For this review, take the finished solid that the model builds, in its own axes (mm). Face numbers are marked on the shaded views. A direction names the side the tool comes from. Coordinates: 2 decimals unless noted, no trailing zeros. Write each loop counter-clockwise with the first axis right and the second up, starting at its lowest first coordinate (ties: lowest second). Pieces come first, ordered by that corner, then holes.
```python
from build123d import *

# Parameters (mm, degrees)
SKETCH1_R           = 5
BOSS_EXTRUDE1_DEPTH = 20
CUT_EXTRUDE2_DEPTH  = 5
CUT_EXTRUDE3_DEPTH  = 1
CUT_EXTRUDE4_DEPTH  = 5
CUT_EXTRUDE5_DEPTH  = 1


with BuildPart() as part:
    # Sketch1 → Boss-Extrude1 (new body)
    with BuildSketch(Plane(origin=(0, 0, 0), x_dir=(1, 0, 0), z_dir=(0, 1, 0))):
        with BuildLine():
            Line((0, 10), (35, 10))
            ThreePointArc((35, 10), (45, 0), (35, -10))
            Line((35, -10), (0, -10))
            ThreePointArc((0, -10), (-10, 0), (0, 10))
        make_face()
        with Locations((35, 0)):
            Circle(SKETCH1_R, mode=Mode.SUBTRACT)
        Polygon((0, 5), (-4.330127, 2.5), (-4.330127, -2.5), (0, -5), (4.330127, -2.5), (4.330127, 2.5), align=None, mode=Mode.SUBTRACT)
    extrude(amount=BOSS_EXTRUDE1_DEPTH)

    # Sketch2 → Cut-Extrude2 (cut)
    with BuildSketch(Plane(origin=(0, 20, 0), x_dir=(1, 0, 0), z_dir=(0, 1, 0))):
        with BuildLine():
            Line((0, 10), (35, 10))
            ThreePointArc((35, 10), (25, 0), (35, -10))
            Line((35, -10), (0, -10))
            ThreePointArc((0, -10), (10, 0), (0, 10))
        make_face()
    extrude(amount=-CUT_EXTRUDE2_DEPTH, mode=Mode.SUBTRACT)

    # Sketch3 → Cut-Extrude3 (cut)
    with BuildSketch(Plane(origin=(0, 15, 0), x_dir=(1, 0, 0), z_dir=(0, 1, 0))):
        with BuildLine():
            Line((26.339746, 5), (8.660254, 5))
            ThreePointArc((8.660254, 5), (10, 0), (8.660254, -5))
            Line((8.660254, -5), (26.339746, -5))
            ThreePointArc((26.339746, -5), (25, 0), (26.339746, 5))
        make_face()
    extrude(amount=-CUT_EXTRUDE3_DEPTH, mode=Mode.SUBTRACT)

    # Sketch4 → Cut-Extrude4 (cut)
    with BuildSketch(Plane.XZ):
        with BuildLine():
            ThreePointArc((0, -10), (5, -8.660254), (8.660254, -5))
            ThreePointArc((8.660254, -5), (10, 0), (8.660254, 5))
            ThreePointArc((8.660254, 5), (5, 8.660254), (0, 10))
            Line((0, 10), (35, 10))
            ThreePointArc((35, 10), (30, 8.660254), (26.339746, 5))
            ThreePointArc((26.339746, 5), (25, 0), (26.339746, -5))
            ThreePointArc((26.339746, -5), (30, -8.660254), (35, -10))
            Line((35, -10), (0, -10))
        make_face()
    extrude(amount=-CUT_EXTRUDE4_DEPTH, mode=Mode.SUBTRACT)

    # Sketch5 → Cut-Extrude5 (cut)
    with BuildSketch(Plane.XZ.offset(-5)):
        with BuildLine():
            ThreePointArc((8.660254, 5), (10, 0), (8.660254, -5))
            Line((8.660254, -5), (26.339746, -5))
            ThreePointArc((26.339746, -5), (25, 0), (26.339746, 5))
            Line((26.339746, 5), (8.660254, 5))
        make_face()
    extrude(amount=-CUT_EXTRUDE5_DEPTH, mode=Mode.SUBTRACT)


solid = part.part
```
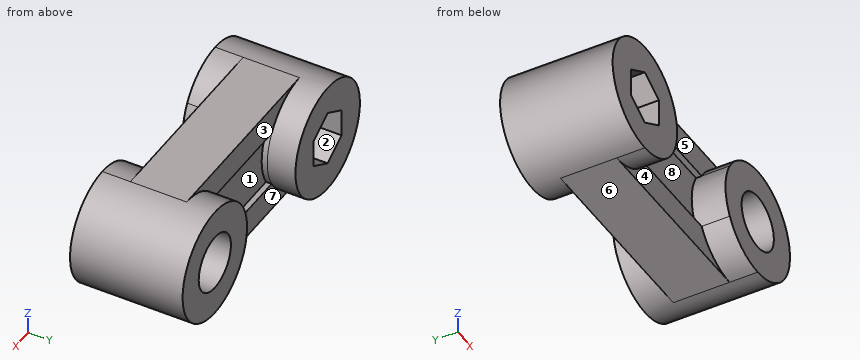
1) For L1, parallel to X at y = 7.75, z = 0; L2, parallel to Z at x = 35, y = 4.25; L3, parallel to X at y = 5.25, z = -3.75, list the stretches that pass through material, from the lowest coordinate up.
2) Tool access review of the marked faces 1, 2, 3, 4 and 5: name each direction out of +Z, -Z, +X, -X, +Y, -Y from which nothing blocks a thin tool from reaching the whole face with its end or side.
3) Consider section B-B (z = 0). Give the boundary of the cut face in (x, y), then the cut area to 3 significant figures.
4) Consider section C-C (y = 8). Give the boundary of the cut face in (x, z), then the cut area to 3 significant figures.
5) Consider section A-A (y = 2.75). Give the boundary of the cut face in (x, z).
6) The part is to be moulded in two halves that separate along Z. For the marked faces 6, 7 and 8, say which applies: pulls with the +Z half, pulls with the -Z half, needs draft (parallel to the pull), parting line crosses it, or undercut.
7) Consider section D-D (x = 38). Give the boundary of the cut face in (y, z).
8) Clearance check with flat-ended pins moving along their axes: P1, Ø3, axis at y = 6, z = 5, coming from the +X side; P2, Ø2.5, axis at x = 13.5, z = -6.5, coming from the +Y side; P3, Ø4, axis at x = 10.5, z = 8, coming from the -Y side. State where each tip first meets the part, or that it passes through.
Results:
1. L1: x = -10 to -4.33, 4.33 to 30, 40 to 45
1. L2: z = -10 to -5, 5 to 10
1. L3: x = -9.27 to -2.17, 2.17 to 9.27, 25.73 to 31.69, 38.31 to 44.27
2. face 1: +Y
2. face 2: +Y, -Y
2. face 3: +Z, +Y
2. face 4: -Z, -Y
2. face 5: +Z, -Y
3. outline: (-10, 0) - (-4.33, 0) - (-4.33, 20) - (-10, 20) - close; (4.33, 0) - (10, 0) - (10, 6) - (25, 6) - (25, 0) - (30, 0) - (30, 20) - (25, 20) - (25, 14) - (10, 14) - (10, 20) - (4.33, 20) - close; (40, 0) - (45, 0) - (45, 20) - (40, 20) - close
3. area: 547 mm2
4. outline: (0, -10) - (35, -10) arc R10 ccw to (35, 10) - (0, 10) arc R10 ccw to start; hole (-4.33, -2.5) - (0, -5) - (4.33, -2.5) - (4.33, 2.5) - (0, 5) - (-4.33, 2.5) - close; hole circle Ø10 at (35, 0)
4. area: 871 mm2
5. outline: circle Ø20 at (0, 0); circle Ø20 at (35, 0); hole (-4.33, -2.5) - (0, -5) - (4.33, -2.5) - (4.33, 2.5) - (0, 5) - (-4.33, 2.5) - close; hole circle Ø10 at (35, 0)
6. face 6: pulls with the -Z half
6. face 7: needs draft
6. face 8: undercut
7. outline: (0, -9.54) - (20, -9.54) - (20, -4) - (0, -4) - close; (0, 4) - (20, 4) - (20, 9.54) - (0, 9.54) - close
8. P1: stops at x = 44.37
8. P2: stops at y = 15
8. P3: stops at y = 5
